```python
from build123d import *

# Parameters (mm, degrees)
F0_W           = 60
F0_H           = 35
F0_R           = 2.25
F0_R_2         = 15.1
F1_DEPTH       = 25.65
F3_D           = 5.5
F3_DEPTH       = 35
F3_CBORE_D     = 10
F3_CBORE_DEPTH = 6
F3_TIP         = 1.6523667023
F4_T1_DEPTH    = 51.3668298797
F5_R           = 1


# Not quite as in the source:
# - a fillet or chamfer that OpenCascade refuses, or shapes differently, is made with other operations: its cross-section is extruded or revolved along the edge and cut away or added


with BuildPart() as f1:
    # F0 (on Front) → F1 (new body)
    with BuildSketch(Plane.XZ):
        Rectangle(F0_W, F0_H)
        with Locations((-16.8874953738, -9.75)):
            Circle(F0_R, mode=Mode.SUBTRACT)
        with Locations((16.8874953738, -9.75)):
            Circle(F0_R, mode=Mode.SUBTRACT)
        with Locations((-16.8874953738, 9.75)):
            Circle(F0_R, mode=Mode.SUBTRACT)
        Circle(F0_R_2, mode=Mode.SUBTRACT)
        with Locations((16.8874953738, 9.75)):
            Circle(F0_R, mode=Mode.SUBTRACT)
    extrude(amount=-F1_DEPTH)

    # F3
    with Locations(Plane.XY.offset(17.5)):
        with Locations((-23, 12.825), (23, 12.825)):
            CounterBoreHole(F3_D / 2, F3_CBORE_D / 2, F3_CBORE_DEPTH, depth=F3_DEPTH)
            with Locations((0, 0, -(F3_DEPTH + F3_TIP / 2))):  # 118° drill point
                Cone(0, F3_D / 2, F3_TIP, mode=Mode.SUBTRACT)

    # F4: chamfer of 5 on 2 edges, made by hand

    # F4_s2 → F4_t1 (cut)
    with BuildSketch(Plane.XZ.offset(-38.5084149398)):
        Polygon((25, 17.5), (30, 12.5), (30, 17.5), align=None)
        Polygon((-30, 12.5), (-25, 17.5), (-30, 17.5), align=None)
    extrude(amount=F4_T1_DEPTH, mode=Mode.SUBTRACT)

    # F5
    f5_edges = [f1.edges().sort_by_distance(p)[0] for p in [
        (-15.1, 25.65, 0),
    ]]
    fillet(f5_edges, radius=F5_R)


solid = f1.part
```
Part model, mm, in its own coordinate system. A direction names the side the tool comes from. Round coordinates to 2 decimals unless told otherwise and drop trailing zeros. Loops run counter-clockwise (first coordinate to the right, second up) from the corner with the lowest first, then second, coordinate; pieces in that order, holes last. Notation, with made-up numbers: (38.25, 59.25) -> (51.25, 59.25) arc R21 ccw to (51.25, 80.25) -> close; hole circle Ø6 at (40, 65). An arc over 180 degrees is marked (long way). Use a Markdown table: item, result.
1) Cut at B-B, the plane y = 22.5. List the corners of the cut face in (x, z), and give its area (3 significant figures).
The answers:
| item | result |
|---|---|
| outline | (-30, -17.5) -> (30, -17.5) -> (30, 12.5) -> (25, 17.5) -> (-25, 17.5) -> (-30, 12.5) -> close; hole circle Ø4.5 at (-16.89, -9.75); hole circle Ø4.5 at (-16.89, 9.75); hole circle Ø30.2 at (0, 0); hole circle Ø4.5 at (16.89, -9.75); hole circle Ø4.5 at (16.89, 9.75) |
| area | 1,300 mm2 |
2) Cut at D-D, the plane z = -9.75. State how many separate pieces and enclosed holes the cut face has, and give its area (3 significant figures).
The answers:
| item | result |
|---|---|
| separate pieces | 4 |
| enclosed holes | 2 |
| area | 669 mm2 |
3) Tool access for faces 4 (the cylindrical face through (-15.68, 12.65, -7.85)), 5 (the flat face through (-20, 13, 11.5)): list every direction of +Z, -Z, +X, -X, +Y, -Y with a clear straight run to the whole face (end or side of a thin tool).
The answers:
| item | result |
|---|---|
| face 4 | +Y, -Y |
| face 5 | +Z |
4) Probe line 1 (X direction, y = 10.5, z = 3); line 2 (X direction, y = 18.25, z = 10.5); line 3 (Z direction, x = -16, y = 1). List the from-to ranges inside material, lowest first. Write a range as [from, to].
The answers:
| item | result |
|---|---|
| line 1 | x = [-30, -24.47], [-21.53, -14.8], [14.8, 21.53], [24.47, 30] |
| line 2 | x = [-30, -19.01], [-14.77, -10.85], [10.85, 14.77], [19.01, 30] |
| line 3 | z = [-17.5, -11.82], [-7.68, 7.68], [11.82, 17.5] |
5) Cut at C-C, the plane x = 0. List the corners of the cut face in (y, z).
The answers:
| item | result |
|---|---|
| outline | (0, -17.5) -> (25.65, -17.5) -> (25.65, -16.1) arc R1 ccw to (24.65, -15.1) -> (0, -15.1) -> close; (0, 15.1) -> (24.65, 15.1) arc R1 ccw to (25.65, 16.1) -> (25.65, 17.5) -> (0, 17.5) -> close |
6) Drop a flat-ended pin along its axis: pin 1 Ø10 at (x, z) = (-9, -5.5) entering from +Y. Give the stop position or say it passes through.
The answers:
| item | result |
|---|---|
| pin 1 | stops at y = 25.48 |
7) Cut at A-A, the plane x = 23. List the corners of the cut face in (y, z) (3 decimals), and give its area (3 significant figures).
The answers:
| item | result |
|---|---|
| outline | (0, -17.5) -> (10.075, -17.5) -> (10.075, 11.5) -> (7.825, 11.5) -> (7.825, 17.5) -> (0, 17.5) -> close; (15.575, -17.5) -> (25.65, -17.5) -> (25.65, 17.5) -> (17.825, 17.5) -> (17.825, 11.5) -> (15.575, 11.5) -> close |
| area | 678 mm2 |
8) Pull direction X, two halves, no side cores. Call faces 1 (the flat face through (-28.6, 13, 13.9)), 2 (the flat face through (30, 13, -3)), 3 (the flat face through (20.9, 10.7, 11.5)): pulls with the +X half, pulls with the -X half, needs draft (parallel to the pull), parting line crosses it, or undercut.
The answers:
| item | result |
|---|---|
| face 1 | pulls with the -X half |
| face 2 | pulls with the +X half |
| face 3 | undercut |
